Check sheet for the modelled part. Datum: model origin and axes. Units: mm. A direction names the side the tool comes from. Give positions to 0.01 mm unless a question says otherwise; leave off trailing zeros. Order: outer loops, then holes, each group sorted by start corner. A loop starts at its lowest first (then second) coordinate and runs counter-clockwise, first axis right, second up.
Item 1: Release check for a two-part mould opening along X. For faces 1 (the cylindrical face through (-25.672, -14.446, 4.93)), 2 (the cylindrical face through (-25.672, 16.554, 4.93)), 3 (the flat face through (-40, -1, 60)), 4 (the flat face through (-42, -40, 25)) record: released by +X, released by -X, zero draft, split by the parting line, or undercut.
Item 2: Sectioned sample at D-D on x = -25. Record the boundary of the cut face in (y, z).
Item 3: Gauge pin test, flat end, axial feed: P1, Ø5, axis at x = -10.5, y = 31.5, coming from the +Z side. Record the tip position at first contact, or that the pin passes through.
Item 4: Material ranges on line 1 along Y through (x, z) = (-44.75, 40); line 2 along Z through (x, y) = (-41, 21); line 3 along Y through (x, z) = (-25, 6.75), recorded low to high.
Item 5: Sectioned sample at B-B on z = 49. Record the boundary of the cut face in (x, y), and give its area (3 significant figures).
Item 6: Sectioned sample at C-C on y = 2. Record the boundary of the cut face in (x, z), and give its area (3 significant figures).
Item 7: Sectioned sample at A-A on y = 15.5. Record the boundary of the cut face in (x, z), and give its area (3 significant figures).
Item 8: Access from +Z, -Z, +X, -X, +Y, -Y to the whole of each face (thin tool, end or side, straight path). Record for faces 5 (the flat face through (-20, -1, 10)), 6 (the cylindrical face through (-25.672, 10.554, 4.93)), 7 (the flat face through (-45, 0, 55)).
Autodesk Inventor part; units mm, degrees
ref_plane "YZ Plane" through (0, 0, 0) normal (1, 0, 0) x (0, 1, 0)
ref_plane "XZ Plane" through (0, 0, 0) normal (0, 1, 0) x (-1, 0, 0)
ref_plane "XY Plane" through (0, 0, 0) normal (0, 0, 1) x (1, 0, 0)
sketch "Sketch1" plane through (0, 0, 0) normal (0, 1, 0) x (-1, 0, 0)
  line L0 (0, 0) -> (50, 0)
  line L1 (50, 0) -> (50, 3.3201)
  line L2 (40, 10) -> (0, 10)
  line L3 (0, 10) -> (0, 0)
  line L4 (50, 70) -> (40, 70)
  line L5 (40, 70) -> (40, 10)
  line L6 (50, 3.3201) -> (50, 70)
  dimension "d0" = 50
  dimension "d1" = 70
  dimension "d2" = 10
  dimension "d3" = 10
extrude "Extrusion1" add sketch "Sketch1" along normal mid plane 80
sketch "Sketch2" plane through (-40, -40, 10) normal (1, 0, 0) x (0, 0, -1)
  line L0 (-45, 65) -> (-15, 65)
  line L1 (-15, 65) -> (-15, 15)
  line L2 (-15, 15) -> (-45, 15)
  line L3 (-45, 15) -> (-45, 65)
  line L4 (-60, 80) -> (0, 80)
  line L5 (-60, 0) -> (-60, 80)
  point P0 (10, 40)
  dimension "d6" = 30
  dimension "d7" = 50
  dimension "d8" = 15
  dimension "d9" = 15
extrude "Extrusion2" cut sketch "Sketch2" against normal through all
sketch "Sketch3" plane through (-40, -40, 10) normal (1, 0, 0) x (0, 0, -1)
  circle A0 centre (-30, 74) radius 3.5
  circle A1 centre (-30, 6) radius 3.5
  line L0 (-60, 0) -> (-60, 80)
  line L1 (-60, 80) -> (0, 80)
  point P0 (10, 40)
  dimension "d12" = 7
  dimension "d13" = 7
  dimension "d14" = 30
  dimension "d15" = 68
  dimension "d16" = 6
  dimension "d17" = 30
extrude "Extrusion3" cut sketch "Sketch3" against normal through all
sketch "Sketch4" plane through (0, 40, 0) normal (0, 0, -1) x (-1, 0, 0)
  circle A0 centre (25, -24.5) radius 1.25
  circle A1 centre (25, -30.5) radius 1.25
  circle A2 centre (25, -49.5) radius 1.25
  circle A3 centre (25, -55.5) radius 1.25
  line L0 (0, -80) -> (0, 0)
  line L1 (50, -80) -> (0, -80)
  point P0 (0, -40)
  dimension "d20" = 2.5
  dimension "d21" = 31
  dimension "d22" = 19
  dimension "d23" = 6
  dimension "d24" = 6
  dimension "d25" = 25
  dimension "d26" = 24.5
  dimension "d32" = 2.5
  dimension "d33" = 2.5
  dimension "d34" = 2.5
  dimension "d35" = 55.5
  dimension "d36" = 49.5
extrude "Extrusion4" cut sketch "Sketch4" against normal through all
properties part number "L-bracket"
Report:
1. face 1: undercut
1. face 2: undercut
1. face 3: released by +X
1. face 4: zero draft
2. outline: (-40, 0) - (-16.75, 0) - (-16.75, 10) - (-40, 10) - close; (-14.25, 0) - (-10.75, 0) - (-10.75, 10) - (-14.25, 10) - close; (-8.25, 0) - (8.25, 0) - (8.25, 10) - (-8.25, 10) - close; (10.75, 0) - (14.25, 0) - (14.25, 10) - (10.75, 10) - close; (16.75, 0) - (40, 0) - (40, 10) - (16.75, 10) - close
3. P1: stops at z = 10
4. line 1: y = -40 to -37.5, -30.5 to -25, 25 to 30.5, 37.5 to 40
4. line 2: z = 0 to 25, 55 to 70
4. line 3: y = -40 to -16.75, -14.25 to -10.75, -8.25 to 8.25, 10.75 to 14.25, 16.75 to 40
5. outline: (-50, -40) - (-40, -40) - (-40, -25) - (-50, -25) - close; (-50, 25) - (-40, 25) - (-40, 40) - (-50, 40) - close
5. area: 300 mm2
6. outline: (-50, 0) - (0, 0) - (0, 10) - (-40, 10) - (-40, 25) - (-50, 25) - close; (-50, 55) - (-40, 55) - (-40, 70) - (-50, 70) - close
6. area: 800 mm2
7. outline: (-50, 0) - (-26.25, 0) - (-26.25, 10) - (-40, 10) - (-40, 25) - (-50, 25) - close; (-50, 55) - (-40, 55) - (-40, 70) - (-50, 70) - close; (-23.75, 0) - (0, 0) - (0, 10) - (-23.75, 10) - close
7. area: 775 mm2
8. face 5: +Z, +X, +Y, -Y
8. face 6: +Z, -Z
8. face 7: +X, -X
